Could you check a few things on this drawing? It's one solid part, dimensions in mm from its lowest x, y, z. A direction names the side the tool comes from. Give positions to 0.01 mm unless a question says otherwise; leave off trailing zeros. Loops run counter-clockwise (first coordinate to the right, second up) from the corner with the lowest first, then second, coordinate; pieces in that order, holes last. Notation, with made-up numbers: (39.5, 70.5) - (91.5, 70.5) arc R27 cw to (91.5, 86.5) - close; hole circle Ø10 at (53.25, -32). An arc over 180 degrees is marked (long way). Put each result on its own line as item: value. Start each with the question number.
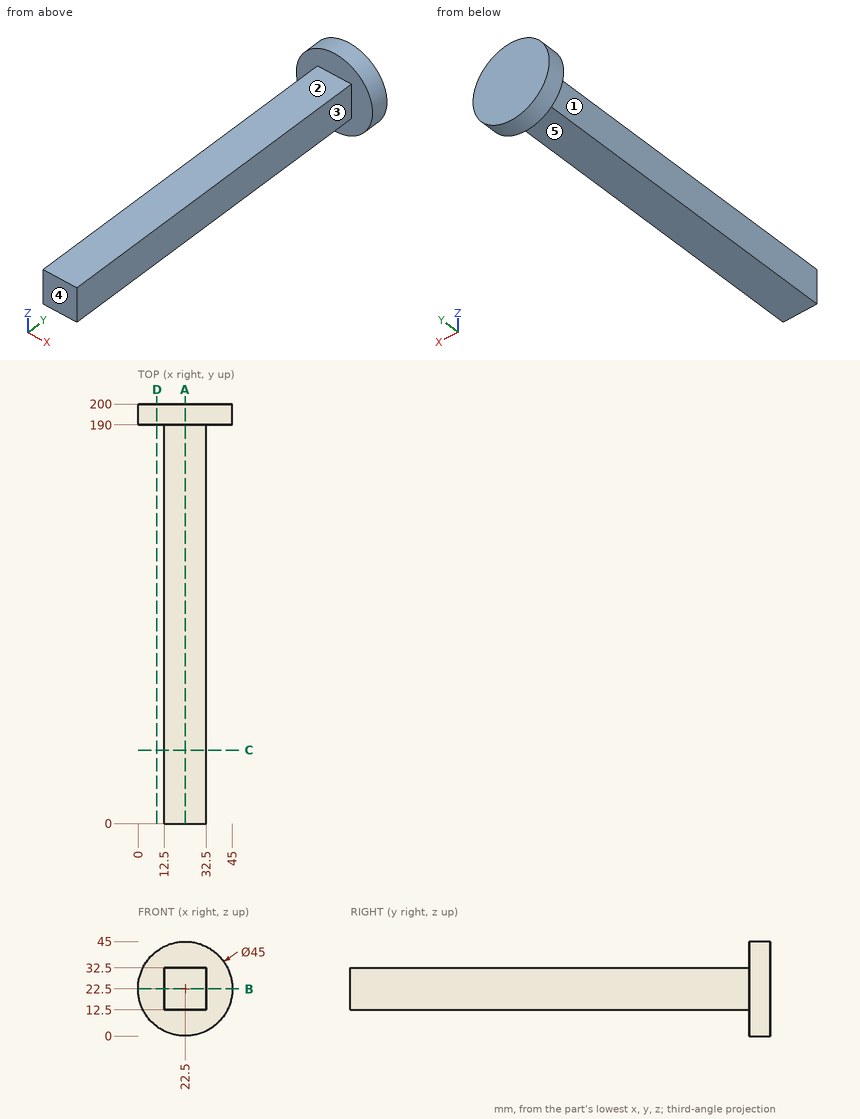
1) Suppose I cut it at A-A on x = 22.5. Please give me the cut outline in (y, z).
2) Suppose I cut it at B-B on z = 22.5. Please give me the cut outline in (x, y).
3) I need wall thicknesses on line 1 (Y direction, x = 8, z = 25.5); line 2 (Z direction, x = 24.5, y = 43.5). Which ranges of each line are inside material? Lowest first, please.
4) Suppose I cut it at C-C on y = 35. Please give me the cut outline in (x, z).
5) Suppose I cut it at D-D on x = 9. Please give me the cut outline in (y, z), plus the area to 3 significant figures.
6) I'm going to push flat-ended pins straight in: P1, Ø3, axis at y = 88.5, z = 23, coming from the -X side; P2, Ø1, axis at x = 11, z = 8, coming from the -Y side; P3, Ø6, axis at x = 23, y = 85.5, coming from the +Z side. Where does each tip first touch, or does it pass through?
7) Which directions (+Z, -Z, +X, -X, +Y, -Y) give clear straight access to the entire face, cutting with the end or side of a thin tool? Please do the marked faces 1, 2, 3, 4 and 5.
Ans:
1. outline: (0, 12.5) - (190, 12.5) - (190, 0) - (200, 0) - (200, 45) - (190, 45) - (190, 32.5) - (0, 32.5) - close
2. outline: (0, 190) - (12.5, 190) - (12.5, 0) - (32.5, 0) - (32.5, 190) - (45, 190) - (45, 200) - (0, 200) - close
3. line 1: y = 190 to 200
3. line 2: z = 12.5 to 32.5
4. outline: (12.5, 12.5) - (32.5, 12.5) - (32.5, 32.5) - (12.5, 32.5) - close
5. outline: (190, 4.5) - (200, 4.5) - (200, 40.5) - (190, 40.5) - close
5. area: 360 mm²
6. P1: stops at x = 12.5
6. P2: stops at y = 190
6. P3: stops at z = 32.5
7. face 1: +Z, -Z, -X, -Y
7. face 2: +Z, +X, -X, -Y
7. face 3: +Z, -Z, +X, -Y
7. face 4: +Z, -Z, +X, -X, -Y
7. face 5: -Z, +X, -X, -Y
